For this review, take the finished solid that the model builds, in its own axes (mm). A direction names the side the tool comes from. Round coordinates to 2 decimals unless told otherwise and drop trailing zeros. Loops run counter-clockwise (first coordinate to the right, second up) from the corner with the lowest first, then second, coordinate; pieces in that order, holes last.
Autodesk Inventor part; units mm, degrees
ref_plane "YZ Plane" through (0, 0, 0) normal (1, 0, 0) x (0, 1, 0)
ref_plane "XZ Plane" through (0, 0, 0) normal (0, 1, 0) x (-1, 0, 0)
ref_plane "XY Plane" through (0, 0, 0) normal (0, 0, 1) x (1, 0, 0)
sketch "Sketch1" plane through (0, 0, 0) normal (0, 1, 0) x (-1, 0, 0)
  line L0 (6, 4.5) -> (-6, 4.5)
  line L1 (-6, 4.5) -> (-6, -4.5)
  line L2 (-6, -4.5) -> (6, -4.5)
  line L3 (6, -4.5) -> (6, 4.5)
  line L4 (6, 4.5) -> (-6, -4.5) construction
  line L5 (-6, 4.5) -> (6, -4.5) construction
  point P0 (0, 0)
  dimension "d4" = 12
  dimension "d5" = 9
extrude "Extrusion1" add sketch "Sketch1" along normal blind 1
sketch "Sketch2" plane through (0, 1, 0) normal (0, 1, 0) x (1, 0, 0)
  point P0 (0, 0)
fillet "Fillet1" radius 1 4 edges at (6, 0.5, 4.5) (6, 0.5, -4.5) (-6, 0.5, -4.5) (-6, 0.5, 4.5)
sketch "Sketch3" plane through (0, 1, 0) normal (0, 1, 0) x (1, 0, 0)
  arc A0 (-6, -3.5) -> (-5, -4.5) centre (-5, -3.5) ccw
  line L0 (-5, -4.5) -> (5, -4.5)
  arc A1 (5, -4.5) -> (6, -3.5) centre (5, -3.5) ccw
  line L1 (6, -3.5) -> (6, 3.5)
  arc A2 (6, 3.5) -> (5, 4.5) centre (5, 3.5) ccw
  line L2 (5, 4.5) -> (-5, 4.5)
  arc A3 (-5, 4.5) -> (-6, 3.5) centre (-5, 3.5) ccw
  line L3 (-6, 3.5) -> (-6, -3.5)
  line L4 (-4.5, -3) -> (4.5, -3)
  line L5 (4.5, -3) -> (4.5, 3)
  line L6 (4.5, 3) -> (-4.5, 3)
  line L7 (-4.5, 3) -> (-4.5, -3)
  point P0 (0, 0)
  dimension "d7" = 1.5
extrude "Extrusion2" cut sketch "Sketch3" against normal up to next contours L7 L6 L5 L4
fillet "Fillet2" radius 1 4 edges at (-4.5, 0.5, 3) (-4.5, 0.5, -3) (4.5, 0.5, 3) (4.5, 0.5, -3)
properties part number "Spacer_3DPrint"
(1) For L1, parallel to X at y = 0.9, z = -1; L2, parallel to Z at x = 2.5, y = 0.8; L3, parallel to X at y = 0.35, z = -2.75, list the stretches that pass through material, from the lowest coordinate up.
(2) Add section B-B (x = 1.75). Give the boundary of the cut face in (y, z).
(3) Add section C-C (y = 0.45). Give the boundary of the cut face in (x, z), plus the area to 3 significant figures.
(4) Add section A-A (z = 0.5). Give the boundary of the cut face in (x, y), plus the area to 3 significant figures.
(5) The part is to be moulded in two halves that separate along Z. For faces 1 (the flat face through (0, 0, 4)), 2 (the cylindrical face through (4.215, 0.493, 2.699)), 3 (the cylindrical face through (5.715, 0.507, -4.199)), 4 (the cylindrical face through (-5.715, 0.507, 4.199)), say which applies: pulls with the +Z half, pulls with the -Z half, needs draft (parallel to the pull), parting line crosses it, or undercut.
(6) For faces 5 (the flat face through (-6, 0.5, 0)), 6 (the cylindrical face through (-4.199, 0.493, 2.715)), list the 3-axis set-ups (+Z, -Z, +X, -X, +Y, -Y) from which the entire face can be reached by the end or side of a thin tool; tool diameter is ignored.
Outcome:
1. L1: x = -6 to -4.5, 4.5 to 6
1. L2: z = -4.5 to -3, 3 to 4.5
1. L3: x = -6 to -4.16, 4.16 to 6
2. outline: (0, -4.5) - (1, -4.5) - (1, -3) - (0, -3) - close; (0, 3) - (1, 3) - (1, 4.5) - (0, 4.5) - close
3. outline: (-6, -3.5) arc R1 ccw to (-5, -4.5) - (5, -4.5) arc R1 ccw to (6, -3.5) - (6, 3.5) arc R1 ccw to (5, 4.5) - (-5, 4.5) arc R1 ccw to (-6, 3.5) - close; hole (-4.5, -2) arc R1 ccw to (-3.5, -3) - (3.5, -3) arc R1 ccw to (4.5, -2) - (4.5, 2) arc R1 ccw to (3.5, 3) - (-3.5, 3) arc R1 ccw to (-4.5, 2) - close
3. area: 54.0 mm2
4. outline: (-6, 0) - (-4.5, 0) - (-4.5, 1) - (-6, 1) - close; (4.5, 0) - (6, 0) - (6, 1) - (4.5, 1) - close
4. area: 3.00 mm2
5. face 1: needs draft
5. face 2: undercut
5. face 3: pulls with the -Z half
5. face 4: pulls with the +Z half
6. face 5: +Z, -Z, -X, +Y, -Y
6. face 6: +Y, -Y
